```python
from build123d import *

# Parameters (mm, degrees)
BOSS_EXTRUDE1_DEPTH            = 1.2
CUT_EXTRUDE1_DEPTH             = 81.831243959
F_2_5_2_5_DIAMETER_HOLE1_D     = 2.5
F_2_5_2_5_DIAMETER_HOLE1_DEPTH = 10
F_2_5_2_5_DIAMETER_HOLE1_TIP   = 0.751075774
HOLEWZD1_AT_2_COUNT            = 2
HOLEWZD1_AT_2_PITCH            = 28.4
HOLEWZD1_AT_3_COUNT            = 2
HOLEWZD1_AT_3_PITCH            = 56.8


with BuildPart() as part:
    # Sketch1 → Boss-Extrude1 (new, symmetric)
    with BuildSketch(Plane.XY):
        Polygon((-24, 0), (24, 0), (37, 21.635633271), (37, 32.5), (-37, 32.5), (-37, 21.635633271), align=None)
    extrude(amount=BOSS_EXTRUDE1_DEPTH, both=True)

    # Sketch2 → Cut-Extrude1 (cut, through all)
    with BuildSketch(Plane(origin=(37, 0, 0), x_dir=(0, 0, -1), z_dir=(1, 0, 0))):
        Polygon((-1.2, 27.883474694), (0.3, 32.5), (-1.2, 32.5), align=None)
    extrude(amount=-CUT_EXTRUDE1_DEPTH, mode=Mode.SUBTRACT)

    # Ø2.5 (2.5) Diameter Hole1
    with Locations(Plane.XY.offset(1.2)):
        with Locations((-7.5, 5.25), (7.5, 5.25)):
            Hole(F_2_5_2_5_DIAMETER_HOLE1_D / 2, depth=F_2_5_2_5_DIAMETER_HOLE1_DEPTH)
            with Locations((0, 0, -(F_2_5_2_5_DIAMETER_HOLE1_DEPTH + F_2_5_2_5_DIAMETER_HOLE1_TIP / 2))):  # 118° drill point
                Cone(0, F_2_5_2_5_DIAMETER_HOLE1_D / 2, F_2_5_2_5_DIAMETER_HOLE1_TIP, mode=Mode.SUBTRACT)

    # Sketch10 → HoleWzd1 (revolve, cut)
    with BuildSketch(Plane(origin=(28.4, 21.2, -1.2), x_dir=(0, 1, 0), z_dir=(1, 0, 0))):
        Polygon((0, 0), (0, 2.4), (1.1, 2.4), (1.1, 2.040774557), (2, 1.5), (2, 0), align=None)
    holewzd1 = revolve(axis=Axis((28.4, 21.2, -7.330023899), (0, 0, 1)), mode=Mode.SUBTRACT)

    # HoleWzd1 at 2: HoleWzd1 ×2
    with Locations(*[(-i * HOLEWZD1_AT_2_PITCH, 0, 0) for i in range(1, HOLEWZD1_AT_2_COUNT)]):
        add(holewzd1, mode=Mode.SUBTRACT)

    # HoleWzd1 at 3: HoleWzd1 ×2
    with Locations(*[(-i * HOLEWZD1_AT_3_PITCH, 0, 0) for i in range(1, HOLEWZD1_AT_3_COUNT)]):
        add(holewzd1, mode=Mode.SUBTRACT)


solid = part.part
```
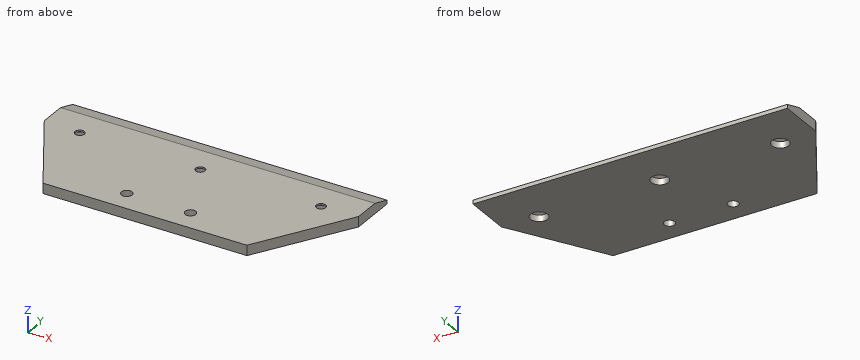
For this review, take the finished solid that the model builds, in its own axes (mm). Give positions to 0.01 mm unless a question says otherwise; leave off trailing zeros. Write each loop counter-clockwise with the first axis right and the second up, starting at its lowest first coordinate (ties: lowest second). Pieces come first, ordered by that corner, then holes. Notation, with made-up numbers: M 16.25,9.25 L 75.25,9.25 A19 cw 75.25,28.25 Z; hole C -1,46.5 d5. An arc over 180 degrees is marked long. Answer as a JSON object with one key per item and string values. Group by question number.
Item 1: For pin 1 Ø3 at (x, y) = (7.5, 5.25) entering from -Z; pin 2 Ø3 at (x, y) = (28.4, 21.2) entering from -Z; pin 3 Ø3.5 at (x, y) = (0, 21.2) entering from -Z; pin 4 Ø2.5 at (x, y) = (-28.4, 21.2) entering from -Z, all flat-tipped, find the tip position at first contact; note any pin that passes through.
Item 2: For probe 1 along X at (y, z) = (21.2, -0.35); probe 2 along X at (y, z) = (5, -0.6); probe 3 along Y at (x, z) = (1, -1.1), list the stretches that pass through material, from the lowest coordinate up. Write a range as [from, to].
Item 3: Consider section A-A on x = 0. Write out the cut boundary in (y, z).
Item 4: Consider section D-D on x = -7.5. Write out the cut boundary in (y, z), plus the area to 3 significant figures.
Item 5: Consider section B-B on y = 5.25. Write out the cut boundary in (x, z).
Item 6: Consider section C-C on x = -20. Write out the cut boundary in (y, z), plus the area to 3 significant figures.
Check result:
{
 "1": {"pin 1": "stops at z = -1.2", "pin 2": "stops at z = 0.6", "pin 3": "stops at z = 0.45", "pin 4": "stops at z = 0.75"},
 "2": {"probe 1": "x = [-36.74, -30.4], [-26.4, -2], [2, 26.4], [30.4, 36.74]", "probe 2": "x = [-27, -8.72], [-6.28, 6.28], [8.72, 27]", "probe 3": "y = [0, 19.47], [22.93, 32.5]"},
 "3": {"outline": "M 0,-1.2 L 19.2,-1.2 L 19.2,0.3 L 20.1,0.84 L 20.1,1.2 L 0,1.2 Z; M 22.3,0.84 L 23.2,0.3 L 23.2,-1.2 L 32.5,-1.2 L 32.5,-0.3 L 27.88,1.2 L 22.3,1.2 Z"},
 "4": {"outline": "M 0,-1.2 L 4,-1.2 L 4,1.2 L 0,1.2 Z; M 6.5,-1.2 L 32.5,-1.2 L 32.5,-0.3 L 27.88,1.2 L 6.5,1.2 Z", "area": "68.5 mm^2"},
 "5": {"outline": "M -27.15,-1.2 L -8.75,-1.2 L -8.75,1.2 L -27.15,1.2 Z; M -6.25,-1.2 L 6.25,-1.2 L 6.25,1.2 L -6.25,1.2 Z; M 8.75,-1.2 L 27.15,-1.2 L 27.15,1.2 L 8.75,1.2 Z"},
 "6": {"outline": "M 0,-1.2 L 32.5,-1.2 L 32.5,-0.3 L 27.88,1.2 L 0,1.2 Z", "area": "74.5 mm^2"}
}
